Source: CAD feature listing. Evaluate the final solid. Frame: model axes, mm. Coordinates: 2 decimals unless noted, no trailing zeros. Order: outer loops, then holes, each group sorted by start corner. A loop starts at its lowest first (then second) coordinate and runs counter-clockwise, first axis right, second up. Notation, with made-up numbers: (29.25, 17) -> (76.25, 17) arc R23 ccw to (76.25, 45) -> close; hole circle Ø10 at (51, 46). An arc over 180 degrees is marked (long way). Put each result on its own line as item: value.
from build123d import *

# Parameters (mm, degrees)
F0_W     = 25.4
F0_H     = 50.8
F1_DEPTH = 25.4
F3_DEPTH = 25.4
F5_DEPTH = 21.59
F6_DEPTH = 25.4


with BuildPart() as f1:
    # F0 (on Front) → F1 (new body, symmetric)
    with BuildSketch(Plane.XZ):
        with Locations((-12.7, 0)):
            Rectangle(F0_W, F0_H)
        with Locations((12.7, 0)):
            Rectangle(F0_W, F0_H)
    extrude(amount=F1_DEPTH, both=True)

    # F2 (on face) → F3 (join)
    with BuildSketch(Plane.XZ.offset(25.4)):
        with BuildLine():
            ThreePointArc((0, -12.7), (-12.7, 0), (0, 12.7))
            Line((0, 12.7), (0, 25.4))
            Line((0, 25.4), (-25.4, 25.4))
            Line((-25.4, 25.4), (-25.4, -25.4))
            Line((-25.4, -25.4), (0, -25.4))
            Line((0, -25.4), (0, -12.7))
        make_face()
        with BuildLine():
            ThreePointArc((0, 12.7), (8.9802561211, 8.9802561211), (12.7, 0))
            ThreePointArc((12.7, 0), (8.9802561211, -8.9802561211), (0, -12.7))
            Line((0, -12.7), (0, -25.4))
            Line((0, -25.4), (25.4, -25.4))
            Line((25.4, -25.4), (25.4, 25.4))
            Line((25.4, 25.4), (0, 25.4))
            Line((0, 25.4), (0, 12.7))
        make_face()
        with BuildLine():
            Line((0, -12.7), (0, 12.7))
            ThreePointArc((0, 12.7), (-12.7, 0), (0, -12.7))
        make_face()
        with BuildLine():
            ThreePointArc((0, -12.7), (8.9802561211, -8.9802561211), (12.7, 0))
            ThreePointArc((12.7, 0), (8.9802561211, 8.9802561211), (0, 12.7))
            Line((0, 12.7), (0, -12.7))
        make_face()
    extrude(amount=F3_DEPTH)

    # F2 (on face) → F4 (revolve, cut)
    with BuildSketch(Plane.XZ.offset(25.4)):
        with BuildLine():
            Line((0, -12.7), (0, 12.7))
            ThreePointArc((0, 12.7), (-12.7, 0), (0, -12.7))
        make_face()
    revolve(axis=Axis((0, -25.4, -7.401805371), (0, 0, -1)), mode=Mode.SUBTRACT)

    # F5 (cut): a face of the model
    f5_faces = [f1.faces().sort_by_distance(p)[0] for p in [
        (0, -50.8, 0),
    ]]
    extrude(f5_faces, amount=-F5_DEPTH, mode=Mode.SUBTRACT)

    # F6 (add): a face of the model
    f6_faces = [f1.faces().sort_by_distance(p)[0] for p in [
        (-24.6815795103, -29.21, 0),
    ]]
    extrude(f6_faces, amount=F6_DEPTH)


solid = f1.part
1. Cut plane B-B on x = 0. Output: boundary loops of the cut face in (y, z), plus the area to 3 significant figures.
Numbers:
outline: (-54.61, -25.4) -> (25.4, -25.4) -> (25.4, 25.4) -> (-54.61, 25.4) -> (-54.61, 12.12) -> (-29.21, 12.12) arc R12.7 cw (long way) to (-29.21, -12.12) -> (-54.61, -12.12) -> close
area: 3,100 mm2
2. Cut plane A-A on z = 0. Output: boundary loops of the cut face in (x, y).
Numbers:
outline: (-25.4, -54.61) -> (-12.12, -54.61) -> (-12.12, -29.21) arc R12.7 cw (long way) to (12.12, -29.21) -> (12.12, -54.61) -> (25.4, -54.61) -> (25.4, 25.4) -> (-25.4, 25.4) -> close
3. First-contact query: pin 1 (22 mm diameter, centred on x = 0, z = 0, fed in from -Y). Flat tip, straight axial feed; report the tip coordinate or a pass-through.
Numbers:
pin 1: stops at y = -19.05
4. Pull-direction query (X, two-part tool) for faces 1 (the cylindrical face through (-10.75, -41.73, -5.59)), 2 (the flat face through (25.4, -14, 0)), 3 (the flat face through (11, -54.61, 6)), 4 (the flat face through (-25.4, -14, 0)); classes: pulls with the +X half, pulls with the -X half, needs draft (parallel to the pull), parting line crosses it, or undercut.
Numbers:
face 1: undercut
face 2: pulls with the +X half
face 3: needs draft
face 4: pulls with the -X half
5. Cut plane C-C on y = -19. Output: boundary loops of the cut face in (x, z), plus the area to 3 significant figures.
Numbers:
outline: (-25.4, -25.4) -> (25.4, -25.4) -> (25.4, 25.4) -> (-25.4, 25.4) -> close; hole circle Ø21.94 at (0, 0)
area: 2,200 mm2
6. Ray query, line 1 along X through (y, z) = (-40, 0); line 2 along X through (y, z) = (-22.5, -1); line 3 along Z through (x, y) = (2, -31.5). Return the intervals inside material, ascending.
Numbers:
line 1: x = -25.4 to -12.12, 12.12 to 25.4
line 2: x = -25.4 to -12.32, 12.32 to 25.4
line 3: z = -25.4 to -11.95, 11.95 to 25.4
